from build123d import *

# Parameters (mm, degrees)
SKETCH1_R           = 9
BOSS_EXTRUDE1_DEPTH = 6


with BuildPart() as part:
    # Sketch1 → Boss-Extrude1 (new body)
    with BuildSketch(Plane.XY):
        with BuildLine():
            Line((-37.5, -9), (-21.265472453, 12))
            Line((-21.265472453, 12), (21.265472453, 12))
            Line((21.265472453, 12), (37.5, -9))
            Line((37.5, -9), (37.5, -80))
            Line((37.5, -80), (3, -80))
            Line((3, -80), (3, -36))
            ThreePointArc((3, -36), (4.060660172, -33.439339828), (1.5, -34.5))
            Line((1.5, -34.5), (-1.5, -34.5))
            ThreePointArc((-1.5, -34.5), (-4.060660172, -33.439339828), (-3, -36))
            Line((-3, -36), (-3, -80))
            Line((-3, -80), (-37.5, -80))
            Line((-37.5, -80), (-37.5, -9))
        make_face()
        Circle(SKETCH1_R, mode=Mode.SUBTRACT)
    extrude(amount=BOSS_EXTRUDE1_DEPTH)


solid = part.part
Verification items for the finished model (mm, model axes). A direction names the side the tool comes from. Give positions to 0.01 mm unless a question says otherwise; leave off trailing zeros. Write each loop counter-clockwise with the first axis right and the second up, starting at its lowest first coordinate (ties: lowest second). Pieces come first, ordered by that corner, then holes. Notation, with made-up numbers: M 18,-12 L 69,-12 A16 cw 69,11 Z; hole C -21,50.25 d10. An arc over 180 degrees is marked long. Write item = value, one per line.
(1) Sectioned sample at A-A (x = 0). Record the cut outline in (y, z).
Found:
outline = M -34.5,0 L -9,0 L -9,6 L -34.5,6 Z; M 9,0 L 12,0 L 12,6 L 9,6 Z
(2) Draft check along Y on faces 1 (the face through (1, -33, 0)), 2 (the face through (4.095, -33.475, 2.958)), 3 (the face through (0, 12, 3)). Enter one of: released by +Y, released by -Y, zero draft, split by the parting line, or undercut.
Found:
face_1 = zero draft
face_2 = undercut
face_3 = released by +Y
(3) Sectioned sample at D-D (x = 29). Record the cut outline in (y, z).
Found:
outline = M -80,0 L 2,0 L 2,6 L -80,6 Z
(4) Material ranges on line 1 (Y direction, x = 0, z = 4.3); line 2 (X direction, y = -34, z = 2.35); line 3 (X direction, y = -59, z = 5.7), recorded low to high.
Found:
line_1 = -34.5 to -9, 9 to 12
line_2 = -37.5 to -4.41, -1.59 to 1.59, 4.41 to 37.5
line_3 = -37.5 to -3, 3 to 37.5
(5) Go/stop test with flat-tipped pins: pin 1 Ø3.5 at (x, z) = (-0.5, 3.5) entering from -Y; pin 2 Ø1 at (x, z) = (28.5, 1.5) entering from +Y. Record where each tip stops, or that it passes through.
Found:
pin_1 = -34.5
pin_2 = 3.29
(6) Access from +Z, -Z, +X, -X, +Y, -Y to the whole of each face (thin tool, end or side, straight path). Record for faces 4 (the face through (3, -58, 3)), 5 (the face through (-37.5, -45, 3)).
Found:
face_4 = +Z, -Z, -Y
face_5 = +Z, -Z, -X, +Y, -Y
(7) Sectioned sample at B-B (z = 1.3). Record the cut outline in (x, y), then the cut area to 3 significant figures.
Found:
outline = M -37.5,-80 L -3,-80 L -3,-36 A1.5 cw long -1.5,-34.5 L 1.5,-34.5 A1.5 cw long 3,-36 L 3,-80 L 37.5,-80 L 37.5,-9 L 21.27,12 L -21.27,12 L -37.5,-9 Z; hole C 0,0 d18
area = 6,020 mm2
(8) Sectioned sample at C-C (y = -42). Record the cut outline in (x, z), then the cut area to 3 significant figures.
Found:
outline = M -37.5,0 L -3,0 L -3,6 L -37.5,6 Z; M 3,0 L 37.5,0 L 37.5,6 L 3,6 Z
area = 414 mm2
